from build123d import *

# Parameters (mm, degrees)
F0_W     = 32
F0_H     = 32
F0_W_2   = 26
F0_H_2   = 26
F1_DEPTH = 100
F2_R     = 25
F2_R_2   = 10
F3_DEPTH = 30


with BuildPart() as f1:
    # F0 (on Top) → F1 (new body)
    with BuildSketch(Plane.XY):
        Rectangle(F0_W, F0_H)
        Rectangle(F0_W_2, F0_H_2, mode=Mode.SUBTRACT)
    extrude(amount=-F1_DEPTH)

    # F2 (on Right) → F3 (join, symmetric)
    with BuildSketch(Plane.YZ):
        with Locations((0, 19)):
            Circle(F2_R)
        with Locations((0, 19)):
            Circle(F2_R_2, mode=Mode.SUBTRACT)
    extrude(amount=F3_DEPTH, both=True)


solid = f1.part
Part model, mm, in its own coordinate system. A direction names the side the tool comes from. Give positions to 0.01 mm unless a question says otherwise; leave off trailing zeros. Loops run counter-clockwise (first coordinate to the right, second up) from the corner with the lowest first, then second, coordinate; pieces in that order, holes last. Notation, with made-up numbers: M 68,-37 L 73,-37 A22 cw 73,-6 Z; hole C 17.25,39 d10. An arc over 180 degrees is marked long. Put each result on its own line as item: value. Start each with the question number.
1) Saw through at D-D (z = -29). List the corners of the cut face in (x, y), then the cut area to 3 significant figures.
2) Saw through at C-C (x = -5.5). List the corners of the cut face in (y, z).
3) 3-axis set-ups, long thin cutter, end or side, ignore diameter. For faces 1 (the flat face through (0, -16, -49)), 2 (the flat face through (0, 16, -49)), 3 (the flat face through (0, 13, -50)): which of +Z, -Z, +X, -X, +Y, -Y reach the whole face in a straight line?
4) Saw through at A-A (z = 19). List the corners of the cut face in (x, y).
5) Pull direction X, two halves, no side cores. Call faces 4 (the flat face through (14, 0, -100)), 5 (the flat face through (16, 0, -49)), 6 (the cylindrical face through (0, 0, -6)): +X half, -X half, draft (parallel to the pull), parting line (faces both ways), or undercut.
6) Probe probe 1 along X at (y, z) = (9, -50.5); probe 2 along Y at (x, z) = (15.5, -78). List the from-to ranges inside material, lowest first.
7) Saw through at B-B (y = 0). List the corners of the cut face in (x, z).
8) Flat gauge pins, fed straight in: pin 1 (16 mm diameter, centred on x = 0, z = -66.5, fed in from -Y); pin 2 (10 mm diameter, centred on x = 21, y = 19, fed in from +Z); pin 3 (8 mm diameter, centred on y = -2, z = -28, fed in from -X). Where does each tip first touch, or does it go through?
Numbers:
1. outline: M -16,-16 L 16,-16 L 16,16 L -16,16 Z; hole M -13,-13 L 13,-13 L 13,13 L -13,13 Z
1. area: 348 mm^2
2. outline: M -16,-100 L -13,-100 L -13,-2.35 A25 ccw 13,-2.35 L 13,-100 L 16,-100 L 16,-0.21 A25 ccw long -16,-0.21 Z; hole C 0,19 d20
3. face 1: -Z, +X, -X, -Y
3. face 2: -Z, +X, -X, +Y
3. face 3: -Z
4. outline: M -30,-25 L 30,-25 L 30,-10 L -30,-10 Z; M -30,10 L 30,10 L 30,25 L -30,25 Z
5. face 4: draft
5. face 5: +X half
5. face 6: undercut
6. probe 1: -16 to -13, 13 to 16
6. probe 2: -16 to 16
7. outline: M -30,-6 L -16,-6 L -16,-100 L -13,-100 L -13,-6 L 13,-6 L 13,-100 L 16,-100 L 16,-6 L 30,-6 L 30,9 L -30,9 Z; M -30,29 L 30,29 L 30,44 L -30,44 Z
8. pin 1: y = -16
8. pin 2: z = 39.71
8. pin 3: x = -16
